Can you work these out from the model? Positions are in its coordinate system, mm. Round coordinates to 2 decimals unless told otherwise and drop trailing zeros. Loops run counter-clockwise (first coordinate to the right, second up) from the corner with the lowest first, then second, coordinate; pieces in that order, holes last. Notation, with made-up numbers: (1.5, 10) -> (53.5, 10) arc R21 ccw to (53.5, 37) -> close; hole circle Ø10 at (22, -25.5). An arc over 180 degrees is marked (long way). Use a Markdown table: item, result.
from build123d import *

# Parameters (mm, degrees)
EXTRUDE_1_DEPTH     = 600
SKETCH_2_R          = 3.25
CUT_EXTRUDE_1_DEPTH = 5.3
SKETCH_3_R          = 2.25
CUT_EXTRUDE_2_DEPTH = 601.125270256
SKETCH1_W           = 15
SKETCH1_H           = 250
CUT_EXTRUDE1_DEPTH  = 100


with BuildPart() as part:
    # Model → Бобышка-Вытянуть1 (new body)
    with BuildSketch(Plane.XY):
        with BuildLine():
            Line((6.8, 0), (7.5, 0.7))
            Line((7.5, 0.7), (7.5, 3.6994391))
            Line((7.5, 3.6994391), (4.7998047, 6.3996344))
            Line((4.7998047, 6.3996344), (4.7998047, 8.409149262))
            Line((4.7998047, 8.409149262), (5.20075838, 8.810103152))
            ThreePointArc((5.20075838, 8.810103152), (5.668922208, 9.789261508), (6.648080611, 10.257425237))
            Line((6.648080611, 10.257425237), (7.5, 11.109345046))
            Line((7.5, 11.109345046), (7.5, 12.449454443))
            Line((7.5, 12.449454443), (6.634490912, 13.314965186))
            ThreePointArc((6.634490912, 13.314965186), (5.668922174, 13.781617126), (5.202270193, 14.747185846))
            Line((5.202270193, 14.747185846), (4.949456226, 15))
            Line((4.949456226, 15), (-4.949456226, 15))
            Line((-4.949456226, 15), (-5.202270193, 14.747185846))
            ThreePointArc((-5.202270193, 14.747185846), (-5.668922174, 13.781617126), (-6.634490912, 13.314965186))
            Line((-6.634490912, 13.314965186), (-7.5, 12.449454443))
            Line((-7.5, 12.449454443), (-7.5, 11.109345046))
            Line((-7.5, 11.109345046), (-6.648080611, 10.257425238))
            ThreePointArc((-6.648080611, 10.257425238), (-5.668922208, 9.789261508), (-5.20075838, 8.810103152))
            Line((-5.20075838, 8.810103152), (-4.7998047, 8.409149262))
            Line((-4.7998047, 8.409149262), (-4.7998047, 6.3996344))
            Line((-4.7998047, 6.3996344), (-7.5, 3.6994391))
            Line((-7.5, 3.6994391), (-7.5, 0.7))
            Line((-7.5, 0.7), (-6.8, 0))
            Line((-6.8, 0), (6.8, 0))
        make_face()
    extrude(amount=EXTRUDE_1_DEPTH)

    # Эскиз2 → Вырез-Вытянуть1 (cut)
    with BuildSketch(Plane(origin=(0, 15, 0), x_dir=(1, 0, 0), z_dir=(0, 1, 0))):
        with Locations(Location((0, -30, 0), (0, 0, 180))):
            Circle(SKETCH_2_R)
        with Locations(Location((0, -90, 0), (0, 0, 180))):
            Circle(SKETCH_2_R)
        with Locations(Location((0, -150, 0), (0, 0, 180))):
            Circle(SKETCH_2_R)
        with Locations(Location((0, -210, 0), (0, 0, 180))):
            Circle(SKETCH_2_R)
        with Locations(Location((0, -270, 0), (0, 0, 180))):
            Circle(SKETCH_2_R)
        with Locations(Location((0, -330, 0), (0, 0, 180))):
            Circle(SKETCH_2_R)
        with Locations(Location((0, -390, 0), (0, 0, 180))):
            Circle(SKETCH_2_R)
        with Locations(Location((0, -450, 0), (0, 0, 180))):
            Circle(SKETCH_2_R)
        with Locations(Location((0, -510, 0), (0, 0, 180))):
            Circle(SKETCH_2_R)
        with Locations(Location((0, -570, 0), (0, 0, 180))):
            Circle(SKETCH_2_R)
    extrude(amount=-CUT_EXTRUDE_1_DEPTH, mode=Mode.SUBTRACT)

    # Эскиз3 → Вырез-Вытянуть2 (cut, through all)
    with BuildSketch(Plane(origin=(0, 9.7, 0), x_dir=(1, 0, 0), z_dir=(0, 1, 0))):
        with Locations(Location((0, -30, 0), (0, 0, 180))):
            Circle(SKETCH_3_R)
        with Locations(Location((0, -90, 0), (0, 0, 180))):
            Circle(SKETCH_3_R)
        with Locations(Location((0, -150, 0), (0, 0, 180))):
            Circle(SKETCH_3_R)
        with Locations(Location((0, -210, 0), (0, 0, 180))):
            Circle(SKETCH_3_R)
        with Locations(Location((0, -270, 0), (0, 0, 180))):
            Circle(SKETCH_3_R)
        with Locations(Location((0, -330, 0), (0, 0, 180))):
            Circle(SKETCH_3_R)
        with Locations(Location((0, -390, 0), (0, 0, 180))):
            Circle(SKETCH_3_R)
        with Locations(Location((0, -450, 0), (0, 0, 180))):
            Circle(SKETCH_3_R)
        with Locations(Location((0, -510, 0), (0, 0, 180))):
            Circle(SKETCH_3_R)
        with Locations(Location((0, -570, 0), (0, 0, 180))):
            Circle(SKETCH_3_R)
    extrude(amount=-CUT_EXTRUDE_2_DEPTH, mode=Mode.SUBTRACT)

    # Sketch1 → Cut-Extrude1 (cut)
    with BuildSketch(Plane(origin=(0, 15, 0), x_dir=(1, 0, 0), z_dir=(0, 1, 0))):
        with Locations((0, -125)):
            Rectangle(SKETCH1_W, SKETCH1_H)
    extrude(amount=-CUT_EXTRUDE1_DEPTH, mode=Mode.SUBTRACT)


solid = part.part
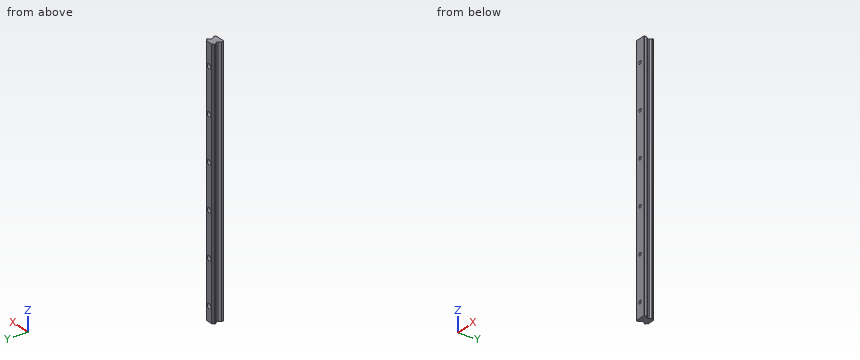
1. I want a section at A-A (z = 525.5). Please give me the cut outline in (x, y).
Answer sheet:
| item | result |
|---|---|
| outline | (-7.5, 0.7) -> (-6.8, 0) -> (6.8, 0) -> (7.5, 0.7) -> (7.5, 3.7) -> (4.8, 6.4) -> (4.8, 8.41) -> (5.2, 8.81) arc R1.63 cw to (6.65, 10.26) -> (7.5, 11.11) -> (7.5, 12.45) -> (6.63, 13.31) arc R1.63 cw to (5.2, 14.75) -> (4.95, 15) -> (-4.95, 15) -> (-5.2, 14.75) arc R1.63 cw to (-6.63, 13.31) -> (-7.5, 12.45) -> (-7.5, 11.11) -> (-6.65, 10.26) arc R1.63 cw to (-5.2, 8.81) -> (-4.8, 8.41) -> (-4.8, 6.4) -> (-7.5, 3.7) -> close |
2. I need wall thicknesses on line 1 (X direction, y = 3, z = 570); line 2 (X direction, y = 12.25, z = 330.5); line 3 (X direction, y = 4.5, z = 337). Which ranges of each line are inside material? Lowest first, please.
Answer sheet:
| item | result |
|---|---|
| line 1 | x = -7.5 to -2.25, 2.25 to 7.5 |
| line 2 | x = -7.5 to -3.21, 3.21 to 7.5 |
| line 3 | x = -6.7 to 6.7 |
3. Will these pins go through, and if not, where does the flat tip stop? pin 1 Ø1.5 at (y, z) = (7.5, 443.5) entering from +X; pin 2 Ø2 at (x, z) = (1.5, 571.5) entering from +Y; pin 3 Ø1 at (y, z) = (7.5, 402) entering from -X.
Answer sheet:
| item | result |
|---|---|
| pin 1 | stops at x = 4.8 |
| pin 2 | stops at y = 9.7 |
| pin 3 | stops at x = -4.8 |
